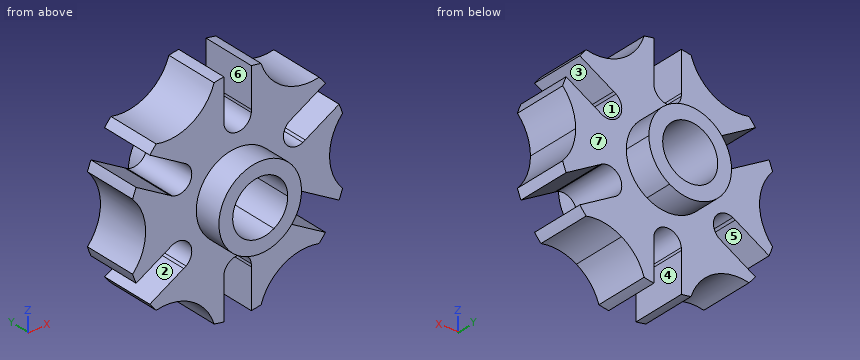
```python
from build123d import *

# Parameters (mm, degrees)
F1_DEPTH = 12.7
F2_DEPTH = 25.4


with BuildPart() as f1:
    # F0 (on Front) → F1 (new body, symmetric)
    with BuildSketch(Plane.XZ):
        with BuildLine():
            ThreePointArc((42.418, 0), (43.966661, 8.270817), (48.402813, 15.421014))
            ThreePointArc((48.402813, 15.421014), (47.655949, 17.594048), (46.811583, 19.731085))
            Line((46.811583, 19.731085), (31.205318, 10.720804))
            ThreePointArc((31.205318, 10.720804), (30.671307, 10.375739), (30.105466, 10.085804))
            ThreePointArc((30.105466, 10.085804), (21.997045, 12.7), (23.787295, 21.029196))
            ThreePointArc((23.787295, 21.029196), (24.321307, 21.374261), (24.887148, 21.664196))
            Line((24.887148, 21.664196), (40.493412, 30.674477))
            ThreePointArc((40.493412, 30.674477), (39.064867, 32.474238), (37.556396, 34.207559))
            ThreePointArc((37.556396, 34.207559), (21.209, 36.735066), (10.846417, 49.628573))
            ThreePointArc((10.846417, 49.628573), (8.591082, 50.068286), (6.31817, 50.405562))
            Line((6.31817, 50.405562), (6.31817, 32.385))
            ThreePointArc((6.31817, 32.385), (6.35, 31.75), (6.31817, 31.115))
            ThreePointArc((6.31817, 31.115), (0, 25.4), (-6.31817, 31.115))
            ThreePointArc((-6.31817, 31.115), (-6.35, 31.75), (-6.31817, 32.385))
            Line((-6.31817, 32.385), (-6.31817, 50.405562))
            ThreePointArc((-6.31817, 50.405562), (-8.591082, 50.068286), (-10.846417, 49.628573))
            ThreePointArc((-10.846417, 49.628573), (-21.209, 36.735066), (-37.556396, 34.207559))
            ThreePointArc((-37.556396, 34.207559), (-39.064867, 32.474238), (-40.493412, 30.674477))
            Line((-40.493412, 30.674477), (-23.787295, 21.029196))
            ThreePointArc((-23.787295, 21.029196), (-21.997045, 12.7), (-30.105466, 10.085804))
            ThreePointArc((-30.105466, 10.085804), (-30.671307, 10.375739), (-31.205318, 10.720804))
            Line((-31.205318, 10.720804), (-46.811583, 19.731085))
            ThreePointArc((-46.811583, 19.731085), (-47.655949, 17.594048), (-48.402813, 15.421014))
            ThreePointArc((-48.402813, 15.421014), (-42.418, 0), (-48.402813, -15.421014))
            ThreePointArc((-48.402813, -15.421014), (-47.655949, -17.594048), (-46.811583, -19.731085))
            Line((-46.811583, -19.731085), (-31.205318, -10.720804))
            ThreePointArc((-31.205318, -10.720804), (-30.671307, -10.375739), (-30.105466, -10.085804))
            ThreePointArc((-30.105466, -10.085804), (-21.997045, -12.7), (-23.787295, -21.029196))
            ThreePointArc((-23.787295, -21.029196), (-24.321307, -21.374261), (-24.887148, -21.664196))
            Line((-24.887148, -21.664196), (-40.493412, -30.674477))
            ThreePointArc((-40.493412, -30.674477), (-39.064867, -32.474238), (-37.556396, -34.207559))
            ThreePointArc((-37.556396, -34.207559), (-21.209, -36.735066), (-10.846417, -49.628573))
            ThreePointArc((-10.846417, -49.628573), (-8.591082, -50.068286), (-6.31817, -50.405562))
            Line((-6.31817, -50.405562), (-6.31817, -32.385))
            ThreePointArc((-6.31817, -32.385), (-6.35, -31.75), (-6.31817, -31.115))
            ThreePointArc((-6.31817, -31.115), (0, -25.4), (6.31817, -31.115))
            ThreePointArc((6.31817, -31.115), (6.35, -31.75), (6.31817, -32.385))
            Line((6.31817, -32.385), (6.31817, -50.405562))
            ThreePointArc((6.31817, -50.405562), (8.591082, -50.068286), (10.846417, -49.628573))
            ThreePointArc((10.846417, -49.628573), (14.820593, -42.211654), (21.209, -36.735066))
            Line((21.209, -36.735066), (9.525, -16.497784))
            ThreePointArc((9.525, -16.497784), (-16.497784, 9.525), (19.05, 0))
            Line((19.05, 0), (42.418, 0))
        make_face()
        with BuildLine():
            ThreePointArc((48.402813, -15.421014), (43.966661, -8.270817), (42.418, 0))
            Line((42.418, 0), (19.05, 0))
            ThreePointArc((19.05, 0), (16.497784, -9.525), (9.525, -16.497784))
            Line((9.525, -16.497784), (21.209, -36.735066))
            ThreePointArc((21.209, -36.735066), (29.146068, -33.940837), (37.556396, -34.207559))
            ThreePointArc((37.556396, -34.207559), (39.064867, -32.474238), (40.493412, -30.674477))
            Line((40.493412, -30.674477), (24.887148, -21.664196))
            ThreePointArc((24.887148, -21.664196), (24.321307, -21.374261), (23.787295, -21.029196))
            ThreePointArc((23.787295, -21.029196), (21.997045, -12.7), (30.105466, -10.085804))
            ThreePointArc((30.105466, -10.085804), (30.671307, -10.375739), (31.205318, -10.720804))
            Line((31.205318, -10.720804), (46.811583, -19.731085))
            ThreePointArc((46.811583, -19.731085), (47.655949, -17.594048), (48.402813, -15.421014))
        make_face()
    extrude(amount=F1_DEPTH, both=True)

    # F0 (on Front) → F2 (join, symmetric)
    with BuildSketch(Plane.XZ):
        with BuildLine():
            ThreePointArc((9.525, -16.497784), (16.497784, -9.525), (19.05, 0))
            Line((19.05, 0), (12.7, 0))
            ThreePointArc((12.7, 0), (10.998523, -6.35), (6.35, -10.998523))
            Line((6.35, -10.998523), (9.525, -16.497784))
        make_face()
        with BuildLine():
            Line((12.7, 0), (19.05, 0))
            ThreePointArc((19.05, 0), (-16.497784, 9.525), (9.525, -16.497784))
            Line((9.525, -16.497784), (6.35, -10.998523))
            ThreePointArc((6.35, -10.998523), (-10.998523, 6.35), (12.7, 0))
        make_face()
    extrude(amount=F2_DEPTH, both=True)


solid = f1.part
```
Here's how the part is built. I have some questions about the finished solid (model axes, mm). Face numbers are marked on the shaded views. A direction names the side the tool comes from. Give positions to 0.01 mm unless a question says otherwise; leave off trailing zeros. Order: outer loops, then holes, each group sorted by start corner. A loop starts at its lowest first (then second) coordinate and runs counter-clockwise, first axis right, second up. Notation, with made-up numbers: (78.5, 79.25) -> (108.5, 79.25) arc R27 cw to (108.5, 108.25) -> close; hole circle Ø5 at (-17.5, 7.5). An arc over 180 degrees is marked (long way). Use CSV: the item, a comma, the result in double quotes. Start each with the question number.
Item 1: Thinking about a two-plate mould opening in X: for the marked faces 1, 2 and 3, which applies, pulls with the +X half, pulls with the -X half, needs draft (parallel to the pull), parting line crosses it, or undercut?
Item 2: On a 3-axis mill with a long thin cutter (end or side, diameter ignored), from which of +Z, -Z, +X, -X, +Y, -Y can I reach the whole of each face in a straight line? I mean the marked faces 4, 5, 6 and 7. Say none if no direction works.
Item 3: Suppose I cut it at A-A (x = 0). List the corners of the cut face in (y, z) for me, and give its area (3 significant figures).
Item 4: Suppose I cut it at B-B (z = -8). List the corners of the cut face in (x, y) for me, and give its area (3 significant figures).
Item 5: I'm going to push flat-ended pins straight in: P1, Ø14.5, axis at y = -5.5, z = -40, coming from the -X side; P2, Ø5, axis at x = 18.5, z = 21.5, coming from the +Y side; P3, Ø10, axis at x = -20.5, z = 21, coming from the -Y side; P4, Ø12, axis at y = -0.5, z = -16, coming from the -X side. Where does each tip first touch, or does it pass through?
Item 6: If I drill on probe 1 along Z at (x, y) = (0, -2); probe 2 along Z at (x, y) = (33.5, 0); probe 3 along Y at (x, z) = (36.5, -33), over which ranges is the centre line in solid material (lowest first)? Write a range as [from, to].
Item 7: Suppose I cut it at C-C (x = 34.5). List the corners of the cut face in (y, z) for me.
Item 8: Suppose I cut it at D-D (y = 18). List the corners of the cut face in (x, z) for me (3 decimals).
Answer block:
1,face 1,"undercut"
1,face 2,"pulls with the -X half"
1,face 3,"pulls with the +X half"
2,face 4,"-Z, +Y, -Y"
2,face 5,"+Y, -Y"
2,face 6,"+Z, +Y, -Y"
2,face 7,"+Y"
3,outline,"(-25.4, -19.05) -> (-12.7, -19.05) -> (-12.7, -25.4) -> (12.7, -25.4) -> (12.7, -19.05) -> (25.4, -19.05) -> (25.4, -12.7) -> (-25.4, -12.7) -> close; (-25.4, 12.7) -> (25.4, 12.7) -> (25.4, 19.05) -> (12.7, 19.05) -> (12.7, 25.4) -> (-12.7, 25.4) -> (-12.7, 19.05) -> (-25.4, 19.05) -> close"
3,area,"968 mm^2"
4,outline,"(-43.86, -12.7) -> (-17.29, -12.7) -> (-17.29, -25.4) -> (-9.86, -25.4) -> (-9.86, 25.4) -> (-17.29, 25.4) -> (-17.29, 12.7) -> (-43.86, 12.7) -> close; (9.86, -25.4) -> (17.29, -25.4) -> (17.29, -12.7) -> (43.86, -12.7) -> (43.86, 12.7) -> (17.29, 12.7) -> (17.29, 25.4) -> (9.86, 25.4) -> close"
4,area,"2,100 mm^2"
5,P1,"stops at x = -38.83"
5,P2,"stops at y = 12.7"
5,P3,"stops at y = -12.7"
5,P4,"stops at x = -48.4"
6,probe 1,"z = [-25.4, -12.7], [12.7, 25.4]"
6,probe 2,"z = [-33.69, -26.64], [-12.05, 12.05], [26.64, 33.69]"
6,probe 3,"y = [-12.7, 12.7]"
7,outline,"(-12.7, -33.75) -> (12.7, -33.75) -> (12.7, -27.21) -> (-12.7, -27.21) -> close; (-12.7, -12.62) -> (12.7, -12.62) -> (12.7, 12.62) -> (-12.7, 12.62) -> close; (-12.7, 27.21) -> (12.7, 27.21) -> (12.7, 33.75) -> (-12.7, 33.75) -> close"
8,outline,"circle Ø38.1 at (0, 0); hole (6.35, -10.999) arc R12.7 ccw to (12.7, 0) arc R12.7 ccw (long way) to start"
